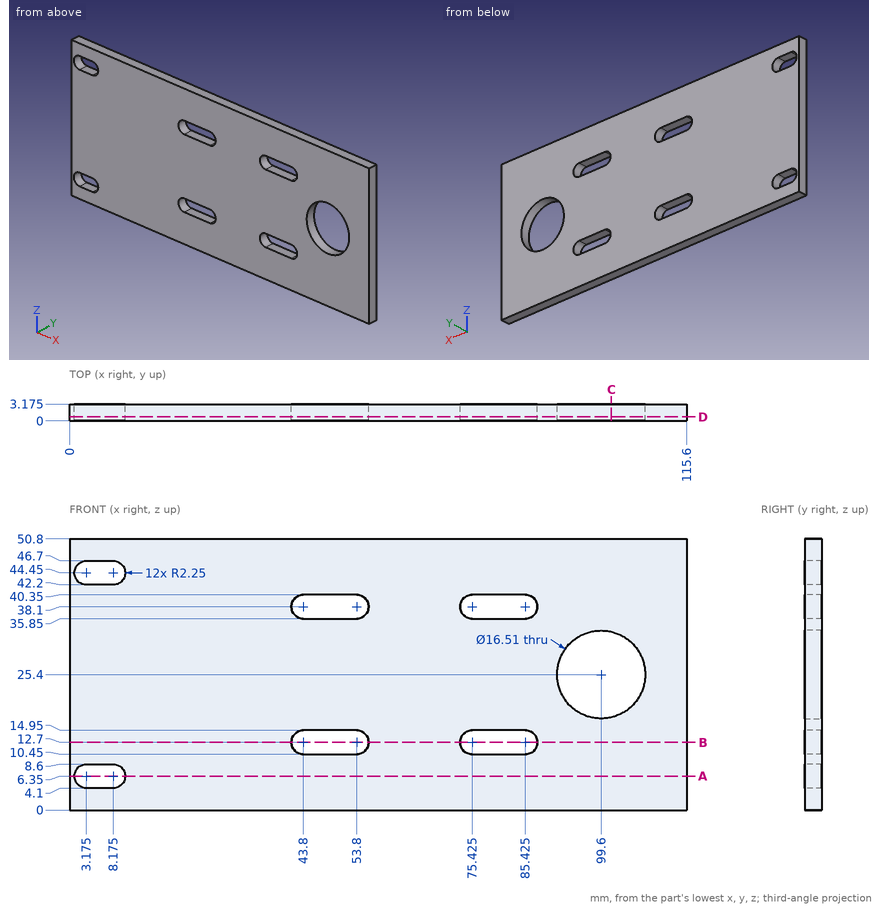
Could you check a few things on this drawing? It's one solid part, dimensions in mm from its lowest x, y, z. Coordinates: 2 decimals unless noted, no trailing zeros. Order: outer loops, then holes, each group sorted by start corner. A loop starts at its lowest first (then second) coordinate and runs counter-clockwise, first axis right, second up.
1) Imagine slicing it at A-A on z = 6.35. List the corners of the cut face in (x, y) for me (3 decimals), and give its area (3 significant figures).
2) Will this pin go through, and if not, where does the flat tip stop? pin 1 (10 mm diameter, centred on x = 99.6, z = 25.4, fed in from +Y).
3) Imagine slicing it at C-C on x = 101.5. List the corners of the cut face in (y, z) for me (3 decimals), and give its area (3 significant figures).
4) I need wall thicknesses on line 1 (Z direction, x = 79.5, y = 1.3); line 2 (X direction, y = 2.05, z = 25.4) (3 decimals); line 3 (X direction, y = 2.8, z = 14). Which ranges of each line are inside material? Lowest first, please.
5) Imagine slicing it at B-B on z = 12.7. List the corners of the cut face in (x, y) for me (3 decimals), and give its area (3 significant figures).
6) Imagine slicing it at D-D on y = 0.75. State how many separate pieces and enclosed holes the cut face has, and give its area (3 significant figures).
Response values:
1. outline: (0, 0) - (0.925, 0) - (0.925, 3.175) - (0, 3.175) - close; (10.425, 0) - (115.6, 0) - (115.6, 3.175) - (10.425, 3.175) - close
1. area: 337 mm2
2. pin 1: passes through
3. outline: (0, 0) - (3.175, 0) - (3.175, 17.367) - (0, 17.367) - close; (0, 33.433) - (3.175, 33.433) - (3.175, 50.8) - (0, 50.8) - close
3. area: 110 mm2
4. line 1: z = 0 to 10.45, 14.95 to 35.85, 40.35 to 50.8
4. line 2: x = 0 to 91.345, 107.855 to 115.6
4. line 3: x = 0 to 41.96, 55.64 to 73.59, 87.26 to 115.6
5. outline: (0, 0) - (41.55, 0) - (41.55, 3.175) - (0, 3.175) - close; (56.05, 0) - (73.175, 0) - (73.175, 3.175) - (56.05, 3.175) - close; (87.675, 0) - (115.6, 0) - (115.6, 3.175) - (87.675, 3.175) - close
5. area: 275 mm2
6. separate pieces: 1
6. enclosed holes: 7
6. area: 5,340 mm2
